Geometry: see drawing. Coordinates: mm, zero at the bounding-box minimum. A direction names the side the tool comes from. Give positions to 0.01 mm unless a question says otherwise; leave off trailing zeros. Write each loop counter-clockwise with the first axis right and the second up, starting at its lowest first coordinate (ties: lowest second). Pieces come first, ordered by that corner, then holes. Notation, with made-up numbers: (25, 26) - (42, 26) arc R15 cw to (42, 41) - close; hole circle Ø6 at (8, 27). An arc over 180 degrees is marked (long way). One line per question, with ' | ' between items. Start each with the question number.
(1) Pin query (flat end, axial travel): pin 1 (4 mm diameter, centred on x = 34, z = 112.5, fed in from -Y). Return the tip coordinate at first contact, or that it passes through.
(2) Access query for the marked faces 1 and 2. Directions: +Z, -Z, +X, -X, +Y, -Y. A direction counts if a zero-diameter tool reaches every point of the face in a straight line with its end or side. Return the directions, or none.
(3) Section C-C, the plane x = 71.5. Return loops of the section in (y, z) (1 decimal), plus the area to 3 significant figures.
(4) Section B-B, the plane z = 33. Return loops of the section in (x, y).
(5) Ray query, line 1 (Z direction, x = 35.5, y = 29) (1 decimal); line 2 (X direction, y = 12, z = 22); line 3 (Y direction, x = 49, z = 125). Return the intervals inside material, ascending. Write a range as [from, to].
(6) Draft query along Z for the marked faces 3, 4 and 5. Return one class per face: +Z half, -Z half, draft (parallel to the pull), parting line (faces both ways), or undercut.
(7) Section A-A, the plane y = 23.5. Return loops of the section in (x, z) (1 decimal).
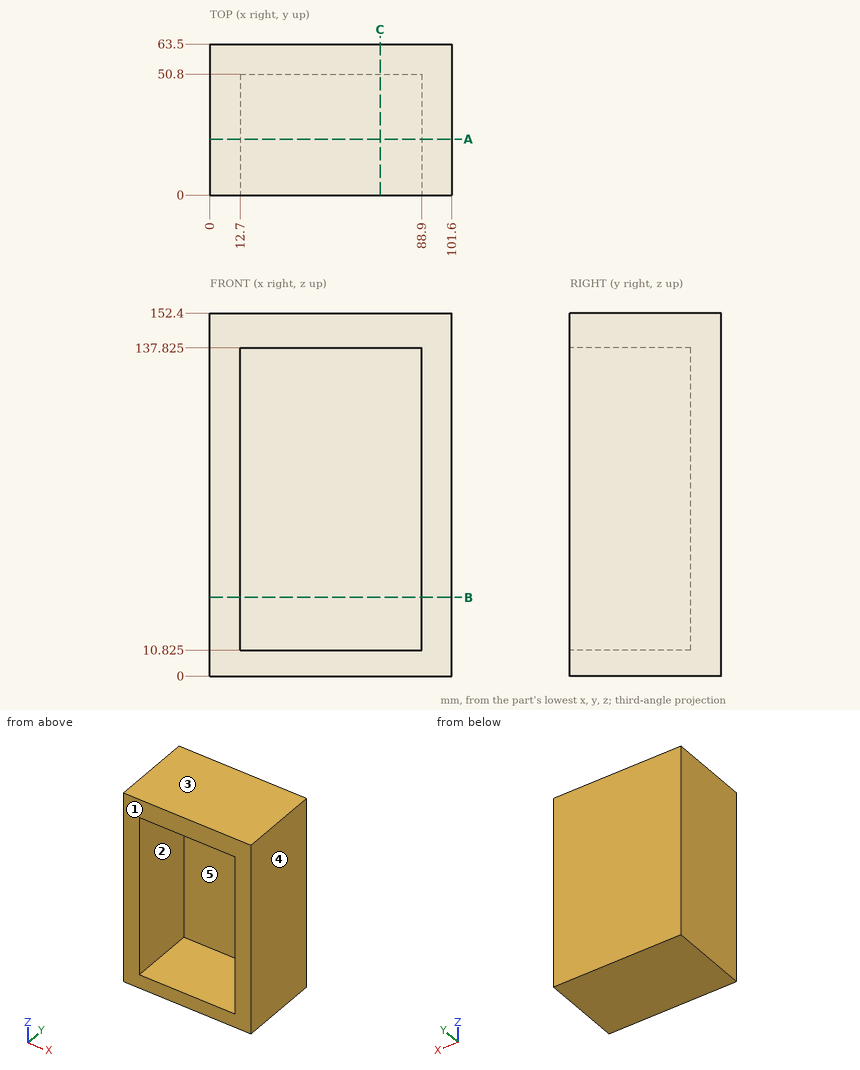
Check sheet entries:
1) pin 1: y = 50.8
2) face 1: +Z, -Z, +X, -X, -Y | face 2: -Y
3) outline: (0, 0) - (63.5, 0) - (63.5, 152.4) - (0, 152.4) - (0, 137.8) - (50.8, 137.8) - (50.8, 10.8) - (0, 10.8) - close | area: 3,230 mm²
4) outline: (0, 0) - (12.7, 0) - (12.7, 50.8) - (88.9, 50.8) - (88.9, 0) - (101.6, 0) - (101.6, 63.5) - (0, 63.5) - close
5) line 1: [0, 10.8], [137.8, 152.4] | line 2: [0, 12.7], [88.9, 101.6] | line 3: [50.8, 63.5]
6) face 3: +Z half | face 4: draft | face 5: undercut
7) outline: (0, 0) - (101.6, 0) - (101.6, 152.4) - (0, 152.4) - close; hole (12.7, 10.8) - (88.9, 10.8) - (88.9, 137.8) - (12.7, 137.8) - close
